Input: part model. Units: mm. Frame: model coordinates. Face numbers are marked on the shaded views. Round coordinates to 2 decimals unless told otherwise and drop trailing zeros. Loops run counter-clockwise (first coordinate to the right, second up) from the corner with the lowest first, then second, coordinate; pieces in that order, holes last.
(1) Draft query along X for the marked faces 1, 2 and 3. Return one class per face: released by +X, released by -X, zero draft, split by the parting line, or undercut.
(2) First-contact query: pin 1 Ø3 at (x, y) = (-12, -2.5) entering from -Z; pin 2 Ø5 at (y, z) = (0, 23) entering from -X; pin 3 Ø3 at (x, y) = (2, 3) entering from -Z; pin 4 Ø5 at (x, y) = (3, -2.5) entering from -Z. Flat tips, straight axial feed; report the tip coordinate or a pass-through.
(3) Line query: line 1 (X direction, y = -0.5, z = -26.5); line 2 (X direction, y = -1.5, z = -18); line 3 (Y direction, x = 10.25, z = 23). Output: solid intervals per line, ascending.
(4) Cut plane D-D, the plane y = 1.5. Give the number of separate pieces and of enclosed holes in the cut face, and give its area (3 significant figures).
(5) Cut plane A-A, the plane z = 23. Output: boundary loops of the cut face in (x, y).
(6) Cut plane C-C, the plane x = -15. Output: boundary loops of the cut face in (y, z).
(7) Cut plane B-B, the plane y = 6.75. Output: boundary loops of the cut face in (x, z), and give its area (4 significant figures).
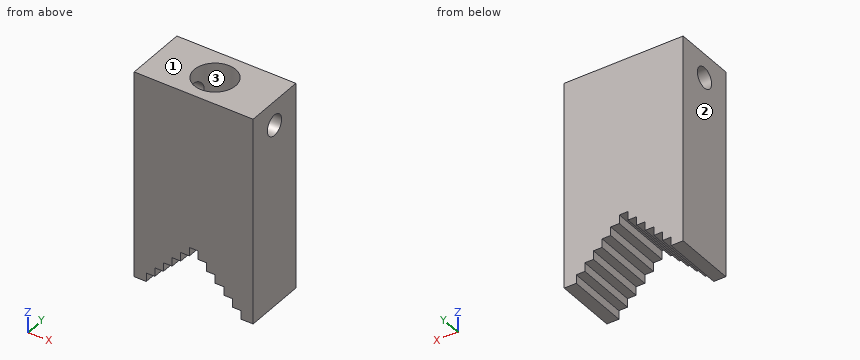
from build123d import *

# Parameters (mm, degrees)
F1_DEPTH = 9
F2_R     = 3
F3_DEPTH = 35


with BuildPart() as f1:
    # F0 (on Front) → F1 (new body, symmetric)
    with BuildSketch(Plane.XZ):
        Polygon((17.25, -30), (17.25, 30), (-17.25, 30), (-17.25, -30), (-13.75, -30), (-13.75, -27.5), (-11.25, -27.5), (-11.25, -25), (-8.75, -25), (-8.75, -22.5), (-6.25, -22.5), (-6.25, -20), (-3.75, -20), (-3.75, -17.5), (-1.25, -17.5), (-1.25, -15), (1.25, -15), (1.25, -17.5), (3.75, -17.5), (3.75, -20), (6.25, -20), (6.25, -22.5), (8.75, -22.5), (8.75, -25), (11.25, -25), (11.25, -27.5), (13.75, -27.5), (13.75, -30), align=None)
    extrude(amount=F1_DEPTH, both=True)

    # F2 (on face) → F3 (cut)
    with BuildSketch(Plane.YZ.offset(17.25)):
        with Locations((0, 23)):
            Circle(F2_R)
    extrude(amount=-F3_DEPTH, mode=Mode.SUBTRACT)

    # F5 (on mid) → F6 (revolve, cut)
    with BuildSketch(Plane.XZ):
        Polygon((0, 30), (-6, 30), (-6, 10), (0, 5.640744832), align=None)
    revolve(axis=Axis((0, 0, 17.820372416), (0, 0, 1)), mode=Mode.SUBTRACT)


solid = f1.part
Reported:
1. face 1: zero draft
1. face 2: released by -X
1. face 3: undercut
2. pin 1: stops at z = -27.5
2. pin 2: passes through
2. pin 3: stops at z = -17.5
2. pin 4: stops at z = -20
3. line 1: x = -17.25 to -11.25, 11.25 to 17.25
3. line 2: x = -17.25 to -3.75, 3.75 to 17.25
3. line 3: y = -9 to -3, 3 to 9
4. separate pieces: 3
4. enclosed holes: 0
4. area: 1,470 mm2
5. outline: (-17.25, -9) - (17.25, -9) - (17.25, -3) - (5.2, -3) arc R6 cw to (-5.2, -3) - (-17.25, -3) - close; (-17.25, 3) - (-5.2, 3) arc R6 cw to (5.2, 3) - (17.25, 3) - (17.25, 9) - (-17.25, 9) - close
6. outline: (-9, -30) - (9, -30) - (9, 30) - (-9, 30) - close; hole circle Ø6 at (0, 23)
7. outline: (-17.25, -30) - (-13.75, -30) - (-13.75, -27.5) - (-11.25, -27.5) - (-11.25, -25) - (-8.75, -25) - (-8.75, -22.5) - (-6.25, -22.5) - (-6.25, -20) - (-3.75, -20) - (-3.75, -17.5) - (-1.25, -17.5) - (-1.25, -15) - (1.25, -15) - (1.25, -17.5) - (3.75, -17.5) - (3.75, -20) - (6.25, -20) - (6.25, -22.5) - (8.75, -22.5) - (8.75, -25) - (11.25, -25) - (11.25, -27.5) - (13.75, -27.5) - (13.75, -30) - (17.25, -30) - (17.25, 30) - (-17.25, 30) - close
7. area: 1,845 mm2
